Source: CAD feature listing. Evaluate the final solid. Frame: model axes, mm. Face numbers are marked on the shaded views. A direction names the side the tool comes from. Coordinates: 2 decimals unless noted, no trailing zeros. Write each loop counter-clockwise with the first axis right and the second up, starting at its lowest first coordinate (ties: lowest second). Pieces come first, ordered by that corner, then holes. Notation, with made-up numbers: M -10.5,72.25 L 31.5,72.25 A25 ccw 31.5,93.25 Z; hole C 89,68 d9. An arc over 180 degrees is marked long. Write item = value, one per line. Start each with the question number.
1. Section query A-A (x = 5). Output: boundary loops of the cut face in (y, z).
2. Line query: line 1 along Y through (x, z) = (-4.5, -0.5); line 2 along Y through (x, z) = (-3.5, 0.25); line 3 along X through (y, z) = (7.5, 3.75). Output: solid intervals per line, ascending.
3. Access query for the marked faces 1 and 2. Directions: +Z, -Z, +X, -X, +Y, -Y. A direction counts if a zero-diameter tool reaches every point of the face in a straight line with its end or side. Return the directions, or none.
4. Section query B-B (y = -6.5). Output: boundary loops of the cut face in (x, z).
5. Pin query (flat end, axial travel): pin 1 Ø1.5 at (y, z) = (-2, 3.5) entering from +X; pin 2 Ø8 at (x, y) = (2, -10) entering from +Z; pin 3 Ø1 at (y, z) = (-1.5, 0) entering from +X. Return the tip coordinate at first contact, or that it passes through.
```python
from build123d import *

# Parameters (mm, degrees)
F1_R     = 1
F5_R     = 1
F9_ANGLE = 30


with BuildPart() as f2:
    # F2: sweep along a path in F0
    with BuildLine(Plane.XY) as f2_path:
        Line((0, 0), (0, -9.0658888221))
        Line((0, -9.0658888221), (-7.5, -16.9975012541))
        Line((-7.5, -16.9975012541), (-7.5, -23.9220938832))
        ThreePointArc((-7.5, -23.9220938832), (-6.0355339059, -27.4576277891), (-2.5, -28.9220938832))
        Line((-2.5, -28.9220938832), (7.5, -28.9220938832))
    # F1 (on Front) → F2 (sweep)
    with BuildSketch(Plane.XZ):
        Circle(F1_R)
    sweep(path=f2_path.line, transition=Transition.RIGHT)

    # F8: sweep along a path in F7
    with BuildLine(Plane.YZ) as f8_path:
        Line((0, 0), (8.6602540378, 5))
    # F5 (on line) → F8 (sweep)
    with BuildSketch(Plane(origin=(0, 0, 0), x_dir=(-1, 0, 0), z_dir=(0, 0.8660254038, 0.5))):
        Circle(F5_R)
    sweep(path=f8_path.line)

    # F3 (on face) → F9 (revolve)
    with BuildSketch(Plane(origin=(0, 0, 0), x_dir=(-1, 0, 0), z_dir=(0, 1, 0))):
        with BuildLine():
            ThreePointArc((-1, 0), (0, -1), (1, 0))
            Line((1, 0), (-1, 0))
        make_face()
    revolve(axis=Axis((0, 0, 0), (1, 0, 0)), revolution_arc=F9_ANGLE)


solid = f2.part
```
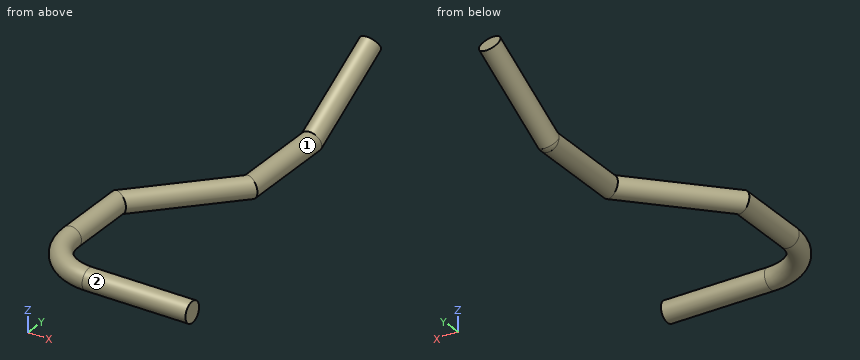
Results are:
q1.outline = C -28.92,0 d2
q2.line_1 = -29.44 to -27.54, -15.09 to -12.56
q2.line_2 = -29.81 to -27.83, -14.18 to -11.36
q2.line_3 = -0.86 to 0.86
q3.face_1 = none
q3.face_2 = +X
q4.outline = C 0,0 d2
q5.pin_1 = through
q5.pin_2 = 1
q5.pin_3 = 1
